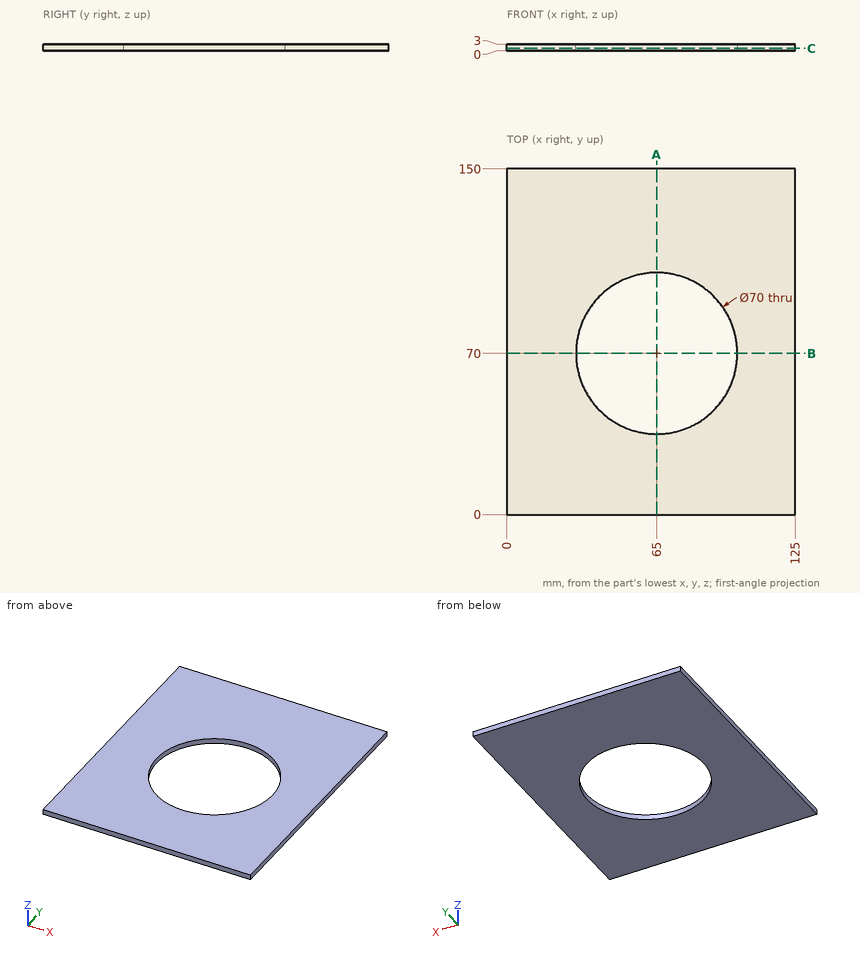
Source: three-view drawing plus pictorial views. Frame: mm from the lowest corner of the part. Round coordinates to 2 decimals unless told otherwise and drop trailing zeros. Loops run counter-clockwise (first coordinate to the right, second up) from the corner with the lowest first, then second, coordinate; pieces in that order, holes last. Notation, with made-up numbers: M 61.5,80 L 92.5,80 A22 cw 92.5,90 Z; hole C 51,7.5 d7. An arc over 180 degrees is marked long. Answer as CSV lines item,"result".
Q1. Line query: line 1 along Y through (x, z) = (65, 1); line 2 along X through (y, z) = (71, 2); line 3 along X through (y, z) = (92, 2.25). Output: solid intervals per line, ascending.
Verdict:
line 1,"y = 0 to 35, 105 to 150"
line 2,"x = 0 to 30.01, 99.99 to 125"
line 3,"x = 0 to 37.78, 92.22 to 125"
Q2. Cut plane C-C (z = 1.1). Return the cut outline in (x, y), plus the area to 3 significant figures.
Verdict:
outline,"M 0,0 L 125,0 L 125,150 L 0,150 Z; hole C 65,70 d70"
area,"14,900 mm^2"
Q3. Cut plane A-A (x = 65). Return the cut outline in (y, z), plus the area to 3 significant figures.
Verdict:
outline,"M 0,0 L 35,0 L 35,3 L 0,3 Z; M 105,0 L 150,0 L 150,3 L 105,3 Z"
area,"240 mm^2"
Q4. Cut plane B-B (y = 70). Return the cut outline in (x, z), plus the area to 3 significant figures.
Verdict:
outline,"M 0,0 L 30,0 L 30,3 L 0,3 Z; M 100,0 L 125,0 L 125,3 L 100,3 Z"
area,"165 mm^2"
